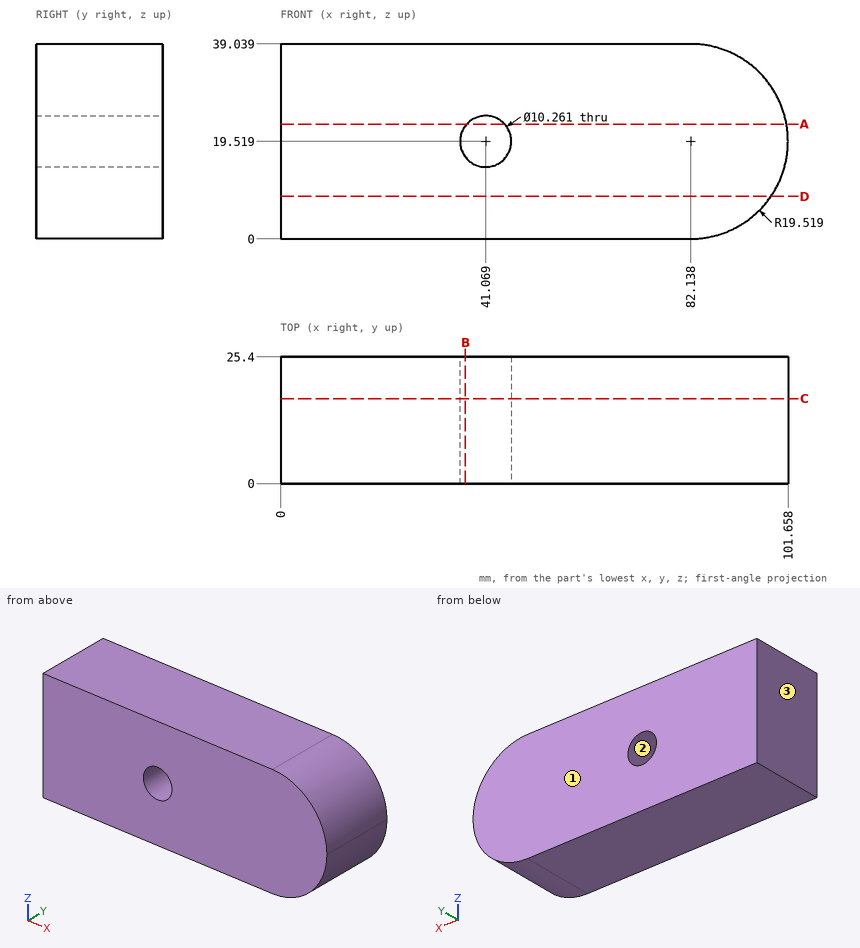
Check sheet for the drawn part. Datum: minimum x, y, z corner. Units: mm. Round coordinates to 2 decimals unless told otherwise and drop trailing zeros. Order: outer loops, then holes, each group sorted by start corner. A loop starts at its lowest first (then second) coordinate and runs counter-clockwise, first axis right, second up. Notation, with made-up numbers: (81.5, 4.25) -> (109.5, 4.25) arc R9 ccw to (109.5, 20.25) -> close; hole circle Ø3 at (60.25, 18.5). An arc over 180 degrees is marked (long way). Return JSON: item names as keys, results as strings. Group by question number.
Q1. Material ranges on probe 1 along X at (y, z) = (18.5, 29); probe 2 along X at (y, z) = (14.5, 37) (1 decimal); probe 3 along Z at (x, y) = (40.5, 2.5), recorded low to high. Write a range as from..to.
Q2. Gauge pin test, flat ends, axial feed: pin 1 (9 mm diameter, centred on x = 41.07, z = 19.52, fed in from +Y); pin 2 (3 mm diameter, centred on y = 15.5, z = 27, fed in from +X). Record the tip position at first contact, or that the pin passes through.
Q3. Release check for a two-part mould opening along X. For the marked faces 1, 2 and 3 record: released by +X, released by -X, zero draft, split by the parting line, or undercut.
Q4. Section check B-B, the plane x = 37. Record the boundary of the cut face in (y, z) (1 decimal), plus the area to 3 significant figures.
Q5. Section check C-C, the plane y = 17. Record the boundary of the cut face in (x, z), plus the area to 3 significant figures.
Q6. Section check A-A, the plane z = 23. Record the boundary of the cut face in (x, y) (1 decimal).
Q7. Section check D-D, the plane z = 8.5. Record the boundary of the cut face in (x, y), plus the area to 3 significant figures.
Numbers:
{
 "1": {"probe 1": "0..99.2", "probe 2": "0..90.8", "probe 3": "0..14.42, 24.62..39.04"},
 "2": {"pin 1": "through", "pin 2": "x = 100.72"},
 "3": {"face 1": "zero draft", "face 2": "undercut", "face 3": "released by -X"},
 "4": {"outline": "(0, 0) -> (25.4, 0) -> (25.4, 16.4) -> (0, 16.4) -> close; (0, 22.6) -> (25.4, 22.6) -> (25.4, 39) -> (0, 39) -> close", "area": "833 mm^2"},
 "5": {"outline": "(0, 0) -> (82.14, 0) arc R19.52 ccw to (82.14, 39.04) -> (0, 39.04) -> close; hole circle Ø10.26 at (41.07, 19.52)", "area": "3,720 mm^2"},
 "6": {"outline": "(0, 0) -> (37.3, 0) -> (37.3, 25.4) -> (0, 25.4) -> close; (44.8, 0) -> (101.3, 0) -> (101.3, 25.4) -> (44.8, 25.4) -> close"},
 "7": {"outline": "(0, 0) -> (98.25, 0) -> (98.25, 25.4) -> (0, 25.4) -> close", "area": "2,500 mm^2"}
}
